Autodesk Inventor part; units mm, degrees
ref_plane "YZ Plane" through (0, 0, 0) normal (1, 0, 0) x (0, 1, 0)
ref_plane "XZ Plane" through (0, 0, 0) normal (0, 1, 0) x (-1, 0, 0)
ref_plane "XY Plane" through (0, 0, 0) normal (0, 0, 1) x (1, 0, 0)
ref_plane "Arbeitsebene1" through (0, 0, 0) normal (0, 0, 1) x (1, 0, 0)
sketch "Skizze1" plane through (0, 0, 0) normal (0, 0, 1) x (1, 0, 0)
  circle A0 centre (0, 0.5522) radius 27.7
  circle A1 centre (0, 0.5522) radius 26.2
  point P0 (0, 0)
  dimension "d11" = 52.4
  dimension "d12" = 55.4
extrude "Extrusion1" add sketch "Skizze1" along normal mid plane 100
sketch "Skizze3" plane through (0, 0, 0) normal (1, 0, 0) x (0, 1, 0)
  line L0 (-27.1478, -50) -> (-27.1478, 50)
  line L1 (28.2522, -50) -> (28.2522, 50)
  line L2 (9.2777, 59.671) -> (-10.7223, 59.671)
  line L3 (-10.7223, 59.671) -> (-10.7223, -5)
  line L4 (-10.7223, -5) -> (9.2777, -5)
  line L5 (9.2777, -5) -> (9.2777, 59.671)
  line L6 (9.2777, 59.671) -> (-10.7223, -5) construction
  line L7 (-10.7223, 59.671) -> (9.2777, -5) construction
  line L8 (0.5522, 50) -> (0.5522, 50)
  point P0 (0, 0)
  point P1 (-0.7223, 27.3355)
  dimension "d13" = 20
  dimension "d14" = 55
extrude "Extrusion3" cut sketch "Skizze3" against normal blind 75
fillet "Rundung1" radius 2 4 edges at (-25.4971, 9.2777, 50) (-25.4971, 9.2777, -5) (-24.4759, -10.7223, 50) (-24.4759, -10.7223, -5)
sketch "Skizze4" plane through (0, 0, 0) normal (1, 0, 0) x (0, 1, 0)
  line L0 (-10.7223, 48) -> (-10.7223, -3)
  line L1 (-8.7223, -5) -> (7.2777, -5)
  line L2 (9.2777, -3) -> (9.2777, 48)
  line L3 (-12.7223, 50) -> (11.2777, 50)
  line L4 (-27.1478, -50) -> (28.2522, -50)
  line L5 (5.5, 35) -> (-5.5, 35)
  line L6 (-7.5, 33) -> (-7.5, 27)
  line L7 (-5.5, 25) -> (5.5, 25)
  line L8 (7.5, 27) -> (7.5, 33)
  line L9 (7.5, 35) -> (-7.5, 25) construction
  line L10 (-7.5, 35) -> (7.5, 25) construction
  line L11 (-25.6478, 50) -> (26.7522, 50)
  line L12 (-2.9499, 34.5) -> (4.0501, 34.5)
  arc A0 (7.5, 33) -> (5.5, 35) centre (5.5, 33) ccw
  arc A1 (-5.5, 35) -> (-7.5, 33) centre (-5.5, 33) ccw
  arc A2 (-7.5, 27) -> (-5.5, 25) centre (-5.5, 27) ccw
  arc A3 (5.5, 25) -> (7.5, 27) centre (5.5, 27) ccw
  point P0 (0, 0)
  point P1 (0, 30)
  dimension "d18" = 15
  dimension "d19" = 10
  dimension "d20" = 15
  dimension "d21" = 2
extrude "Extrusion4" cut sketch "Skizze4" along normal through all
properties part number "Planktoscope_connectortube"
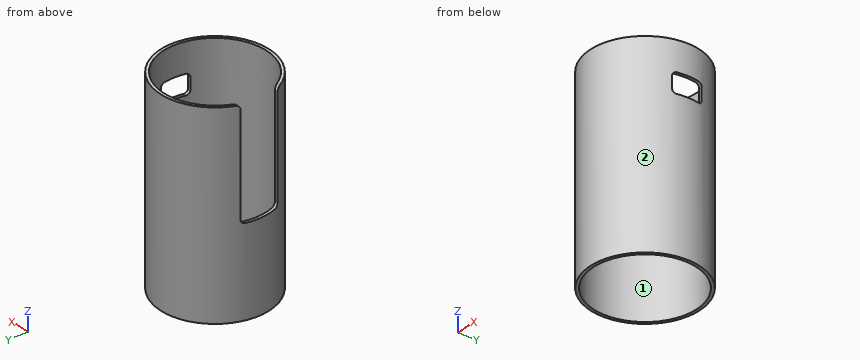
Geometry check sheet. Reference: the model listing, model coordinates, mm. Face numbers are marked on the shaded views. Round coordinates to 2 decimals unless told otherwise and drop trailing zeros. Loops run counter-clockwise (first coordinate to the right, second up) from the corner with the lowest first, then second, coordinate; pieces in that order, holes last. Notation, with made-up numbers: (10.5, 81.5) - (32.5, 81.5) arc R20 cw to (32.5, 93.5) - close; hole circle Ø1 at (-6.5, 46.25). An arc over 180 degrees is marked (long way). Use a Markdown table: item, result.
Q1. Cross-section at B-B on y = -22. Record the cut outline in (x, z), plus the area to 3 significant figures.
Solutions:
| item | result |
|---|---|
| outline | (-16.08, -50) - (-13.34, -50) - (-13.34, 50) - (-16.08, 50) - close; (13.34, -50) - (16.08, -50) - (16.08, 50) - (13.34, 50) - close |
| area | 550 mm2 |
Q2. Go/stop test with flat-tipped pins: P1, Ø1.7, axis at x = 25.5, z = 30.5, coming from the +Y side; P2, Ø10, axis at y = 14.5, z = 2, coming from the +X side (3 decimals); P3, Ø0.8, axis at x = -24.5, z = 27.5, coming from the +Y side; P4, Ø8, axis at x = 19.5, y = 8.5, coming from the -Z side. Record where each tip stops, or that it passes through.
Solutions:
| item | result |
|---|---|
| P1 | stops at y = 13.19 |
| P2 | stops at x = 26.215 |
| P3 | stops at y = 14.21 |
| P4 | passes through |
Q3. Cross-section at C-C on z = -22.5. Record the cut outline in (x, y), plus the area to 3 significant figures.
Solutions:
| item | result |
|---|---|
| outline | circle Ø55.4 at (0, 0.55); hole circle Ø52.4 at (0, 0.55) |
| area | 254 mm2 |
Q4. Cross-section at A-A on x = 0. Record the cut outline in (y, z), plus the area to 3 significant figures.
Solutions:
| item | result |
|---|---|
| outline | (-27.15, -50) - (-25.65, -50) - (-25.65, 50) - (-27.15, 50) - close; (26.75, -50) - (28.25, -50) - (28.25, 50) - (26.75, 50) - close |
| area | 300 mm2 |
Q5. Material ranges on line 1 (Y direction, x = 0, z = -1); line 2 (X direction, y = -23, z = -1); line 3 (Y direction, x = -13, z = 8), recorded low to high.
Solutions:
| item | result |
|---|---|
| line 1 | y = -27.15 to -25.65, 26.75 to 28.25 |
| line 2 | x = -14.58 to -11.48, 11.48 to 14.58 |
| line 3 | y = -23.91 to -22.2, 23.3 to 25.01 |
Q6. Draft check along Y on the marked faces 1 and 2. Enter one of: released by +Y, released by -Y, zero draft, split by the parting line, or undercut.
Solutions:
| item | result |
|---|---|
| face 1 | undercut |
| face 2 | split by the parting line |
Q7. Cross-section at D-D on z = 10. Record the cut outline in (x, y), plus the area to 3 significant figures.
Solutions:
| item | result |
|---|---|
| outline | (-26.29, 9.28) - (-24.7, 9.28) arc R26.2 cw (long way) to (-23.65, -10.72) - (-25.3, -10.72) arc R27.7 ccw (long way) to start |
| area | 223 mm2 |
